```python
from build123d import *

# Parameters (mm, degrees)
F0_W          = 25
F0_H          = 25
F0_W_2        = 19
F0_H_2        = 19
F1_DEPTH      = 12.5
F1_DEPTH_BACK = 12.5
F2_W          = 19
F2_H          = 19
F3_DEPTH      = 25
F3_DEPTH_BACK = 25
F4_W          = 19
F4_H          = 19
F5_DEPTH      = 25
F5_DEPTH_BACK = 25
F6_SIZE       = 0.5
F9_DEPTH      = 5.5355339059


with BuildPart() as f1:
    # F0 (on Front) → F1 (new body, two sides)
    with BuildSketch(Plane.XZ) as f1_sk:
        Rectangle(F0_W, F0_H)
        Rectangle(F0_W_2, F0_H_2, mode=Mode.SUBTRACT)
    extrude(amount=F1_DEPTH)
    extrude(f1_sk.sketch, amount=-F1_DEPTH_BACK)

    # F2 (on Right) → F3 (cut, two sides)
    with BuildSketch(Plane.YZ) as f3_sk:
        Rectangle(F2_W, F2_H)
    extrude(amount=-F3_DEPTH, mode=Mode.SUBTRACT)
    extrude(f3_sk.sketch, amount=F3_DEPTH_BACK, mode=Mode.SUBTRACT)

    # F4 (on Top) → F5 (cut, two sides)
    with BuildSketch(Plane.XY) as f5_sk:
        Rectangle(F4_W, F4_H)
    extrude(amount=-F5_DEPTH, mode=Mode.SUBTRACT)
    extrude(f5_sk.sketch, amount=F5_DEPTH_BACK, mode=Mode.SUBTRACT)

    # F6
    f6_edges = [f1.edges().sort_by_distance(p)[0] for p in [
        (12.5, -12.5, 0),
        (12.5, 0, -12.5),
        (12.5, 0, 12.5),
        (12.5, 12.5, 0),
        (12.5, 0, -9.5),
        (12.5, -9.5, 0),
        (12.5, 0, 9.5),
        (12.5, 9.5, 0),
        (0, -12.5, 12.5),
        (-12.5, 0, 12.5),
        (0, 12.5, 12.5),
        (9.5, 0, 12.5),
        (0, -9.5, 12.5),
        (-9.5, 0, 12.5),
        (0, 9.5, 12.5),
        (0, -12.5, -12.5),
        (-12.5, -12.5, 0),
        (9.5, -12.5, 0),
        (0, -12.5, -9.5),
        (-9.5, -12.5, 0),
        (0, -12.5, 9.5),
        (0, 12.5, -12.5),
        (-12.5, 12.5, 0),
        (9.5, 12.5, 0),
        (0, 12.5, -9.5),
        (-9.5, 12.5, 0),
        (0, 12.5, 9.5),
        (-12.5, 0, -12.5),
        (-12.5, 0, -9.5),
        (-12.5, 9.5, 0),
        (-12.5, 0, 9.5),
        (-12.5, -9.5, 0),
        (9.5, 0, -12.5),
        (0, 9.5, -12.5),
        (-9.5, 0, -12.5),
        (0, -9.5, -12.5),
    ]]
    chamfer(f6_edges, length=F6_SIZE)

    # F8 (on offset) → F9 (join, through all)
    with BuildSketch(Plane(origin=(13.321367205, -13.321367205, -13.321367205), x_dir=(0.8164965809, 0.4082482905, 0.4082482905), z_dir=(0.5773502692, -0.5773502692, -0.5773502692))):
        Polygon((2.9082482905, -4.3301270189), (0.4082482905, 0), (2.9082482905, 4.3301270189), (2.2958758548, 4.6836804095), (-0.2041241452, 0.3535533906), (-5.2041241452, 0.3535533906), (-5.2041241452, -0.3535533906), (-0.2041241452, -0.3535533906), (2.2958758548, -4.6836804095), align=None)
    extrude(amount=-F9_DEPTH)


solid = f1.part
```
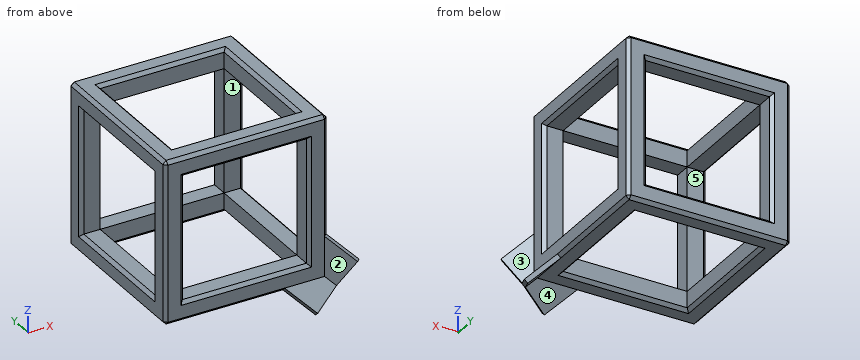
CAD build for the part. Positions are in the model's coordinates, mm. Face numbers are marked on the shaded views. A direction names the side the tool comes from. Coordinates: 2 decimals unless noted, no trailing zeros. Write each loop counter-clockwise with the first axis right and the second up, starting at its lowest first coordinate (ties: lowest second). Pieces come first, ordered by that corner, then holes.
(1) Cut at D-D, the plane y = -11.5. List the corners of the cut face in (x, z).
(2) 3-axis set-ups, long thin cutter, end or side, ignore diameter. For the marked faces 1 and 2: which of +Z, -Z, +X, -X, +Y, -Y reach the whole face in a straight line?
(3) Drill centre line: probe 1 along X at (y, z) = (6.25, 10.75). Where is it in solid material? Low to high.
(4) Two-plate mould, pull along Z, no slides. Class the marked faces 3, 4 and 5: +Z half, -Z half, draft (parallel to the pull), parting line (faces both ways), or undercut.
(5) Cut at C-C, the plane x = 11. List the corners of the cut face in (y, z), and give its area (3 significant figures).
(6) Cut at A-A, the plane x = -8.5. List the corners of the cut face in (y, z).
(7) Flat gauge pins, fed straight in: pin 1 (0.8 mm diameter, centred on y = 0.5, z = -10.5, fed in from +X); pin 2 (10 mm diameter, centred on x = 4.5, z = 6.5, fed in from -Y); pin 3 (1.2 mm diameter, centred on x = 4, y = 10.5, fed in from -Z). Where does each tip first touch, or does it go through?
Geometry says:
1. outline: (-12.5, -12) - (-12, -12.5) - (12, -12.5) - (13.98, -14.48) - (14.48, -13.98) - (12.5, -12) - (12.5, 12) - (12, 12.5) - (-12, 12.5) - (-12.5, 12) - close; hole (-9.5, -9.5) - (9.5, -9.5) - (9.5, 9.5) - (-9.5, 9.5) - close
2. face 1: +X, -X
2. face 2: +Z, -X, -Y
3. probe 1: x = -12.5 to -9.5, 9.5 to 12.5
4. face 3: draft
4. face 4: -Z half
4. face 5: undercut
5. outline: (-14.73, -14.23) - (-14.23, -14.73) - (-12, -12.5) - (12, -12.5) - (12.5, -12) - (12.5, 12) - (12, 12.5) - (-12, 12.5) - (-12.5, 12) - (-12.5, -12) - close; hole (-9.5, -9.5) - (9.5, -9.5) - (9.5, 9.5) - (-9.5, 9.5) - close
5. area: 266 mm2
6. outline: (-12.5, -12) - (-12, -12.5) - (-10, -12.5) - (-9.5, -12) - (-9.5, -9.5) - (-12, -9.5) - (-12.5, -10) - close; (-12.5, 10) - (-12, 9.5) - (-9.5, 9.5) - (-9.5, 12) - (-10, 12.5) - (-12, 12.5) - (-12.5, 12) - close; (9.5, -12) - (10, -12.5) - (12, -12.5) - (12.5, -12) - (12.5, -10) - (12, -9.5) - (9.5, -9.5) - close; (9.5, 9.5) - (12, 9.5) - (12.5, 10) - (12.5, 12) - (12, 12.5) - (10, 12.5) - (9.5, 12) - close
7. pin 1: stops at x = 12.5
7. pin 2: stops at y = -12.5
7. pin 3: stops at z = -12.5
